from build123d import *


with BuildPart() as f1:
    # F0 (on Front) → F1 (revolve)
    with BuildSketch(Plane.XZ):
        Polygon((-63.250169, 65.144755), (-76.658033, 65.144755), (-76.658033, 54.65164), (-77.071565, 30.926656), (-61.379056, 25.757357), (-61.379056, 15.4255), (-82.042769, 15.4255), (-82.042769, -84.449112), (-53.917158, -84.449112), (-53.917158, -121.758595), (-18.071475, -121.758595), (-18.071475, -78.552626), (-42.846885, -70.391312), (-42.846885, -8.307049), (18.071476, 20.257542), (106.680006, 30.167704), (106.800616, 65.144755), (90.154849, 65.144755), (90.154849, 44.741478), (18.405836, 44.741478), (10.369949, 35.515223), (-18.903643, 35.515223), (-32.062296, 44.741478), (-63.250169, 44.741478), align=None)
    revolve(axis=Axis((-35.994316, 0, -121.758595), (-1, 0, 0)))


solid = f1.part
Model file for the job. Use its own axes, mm. A direction names the side the tool comes from. Round coordinates to 2 decimals unless told otherwise and drop trailing zeros. Order: outer loops, then holes, each group sorted by start corner. A loop starts at its lowest first (then second) coordinate and runs counter-clockwise, first axis right, second up.
(1) Band-saw the part on B-B (x = 78). List the corners of the cut face in (y, z), then the cut area to 3 significant figures.
(2) Band-saw the part on A-A (x = 0.5). List the corners of the cut face in (y, z), then the cut area to 3 significant figures.
(3) Pin check, flat tips, straight feed: pin 1 (12 mm diameter, centred on x = -5, z = -220, fed in from -Y); pin 2 (5 mm diameter, centred on x = 48, y = -49, fed in from +Z); pin 3 (3 mm diameter, centred on x = 17.5, y = -26, fed in from +Z). Stop position of each tip, or through.
(4) Pull direction Y, two halves, no side cores. Call faces 1 (the face through (90.155, -110, -247)), 2 (the face through (-42.847, -49, -145)), 3 (the face through (-62.141, 6.497, -269.383)), 4 (the face through (-4.472, -95.699, -246.566)): released by +Y, released by -Y, zero draft, split by the parting line, or undercut.
(5) Drill centre lines: line 1 (Z direction, x = -74, y = -17); line 2 (Z direction, x = -67.5, y = -28.5); line 3 (Y direction, x = 38, z = -149.5). Where is each one in solid material? Low to high.
(6) 3-axis set-ups, long thin cutter, end or side, ignore diameter. For faces 5 (the face through (-63.25, -110, 4)), 6 (the face through (-18.071, 1, -121)), 7 (the face through (-70.05, -71.59, 50.89)), 8 (the face through (-76.658, 112, 16)): which of +Z, -Z, +X, -X, +Y, -Y reach the whole face in a straight line?
Verdict:
1. outline: circle Ø333 at (0, -121.76); hole circle Ø297.44 at (0, -121.76)
1. area: 17,600 mm2
2. outline: circle Ø314.55 at (0, -121.76); hole circle Ø267.55 at (0, -121.76)
2. area: 21,500 mm2
3. pin 1: stops at y = -127.38
3. pin 2: stops at z = 38.12
3. pin 3: stops at z = 42.88
4. face 1: zero draft
4. face 2: undercut
4. face 3: undercut
4. face 4: split by the parting line
5. line 1: z = -307.89 to -272.48, -257.89 to -154.97, -88.55 to 14.37, 28.96 to 64.37
5. line 2: z = -306.48 to -268.55, -255.95 to -145.84, -97.68 to 12.43, 25.03 to 62.96
5. line 3: y = -164.17 to -141.55, 141.55 to 164.17
6. face 5: none
6. face 6: +X
6. face 7: +X, -X
6. face 8: -X
